Autodesk Inventor part; units mm, degrees
ref_plane "YZ Plane" through (0, 0, 0) normal (1, 0, 0) x (0, 1, 0)
ref_plane "XZ Plane" through (0, 0, 0) normal (0, 1, 0) x (-1, 0, 0)
ref_plane "XY Plane" through (0, 0, 0) normal (0, 0, 1) x (1, 0, 0)
sketch "スケッチ1" plane through (0, 0, 0) normal (0, 0, 1) x (1, 0, 0)
  line L0 (0, 0) -> (-22, 0)
  line L1 (-22, 0) -> (-22, 94)
  line L2 (-22, 94) -> (0, 94)
  line L3 (0, 94) -> (0, 0)
  dimension "d0" = 22
  dimension "d1" = 94
extrude "押し出し1" add sketch "スケッチ1" along normal blind 1.5
sketch "スケッチ2" plane through (0, 0, 0) normal (0, 0, -1) x (-1, 0, 0)
  line L0 (5, 24.2) -> (5, 94)
  circle A0 centre (2.5, 84) radius 1.6
  line L1 (0, 94) -> (22, 94)
  line L2 (5, 94) -> (0, 94)
  circle A1 centre (2.5, 59) radius 1.6
  circle A2 centre (2.5, 34) radius 1.6
  circle A3 centre (2.5, 9) radius 1.6
  point P0 (0, 0)
  point P1 (2.5, 94)
  dimension "d4" = 3.2
  dimension "d5" = 10
  dimension "d8" = 25
extrude "押し出し2" cut sketch "スケッチ2" against normal through all
sketch "スケッチ3" plane through (0, 0, 0) normal (0, 0, -1) x (-1, 0, 0)
  line L0 (3.2909, 24.2) -> (5, 24.2)
  line L1 (0, 0) -> (0, 94)
  line L2 (0, 25.2) -> (6, 25.2)
  line L3 (6, 25.2) -> (6, 0)
  line L4 (6, 0) -> (0, 0)
  line L5 (0, 0) -> (0, 25.2)
  line L6 (5, 14.2) -> (5, 24.2)
  line L7 (22, 0) -> (0, 0)
  dimension "d15" = 1
  dimension "d16" = 1
extrude "押し出し3" cut sketch "スケッチ3" against normal through all
properties part number "rail_backcover"
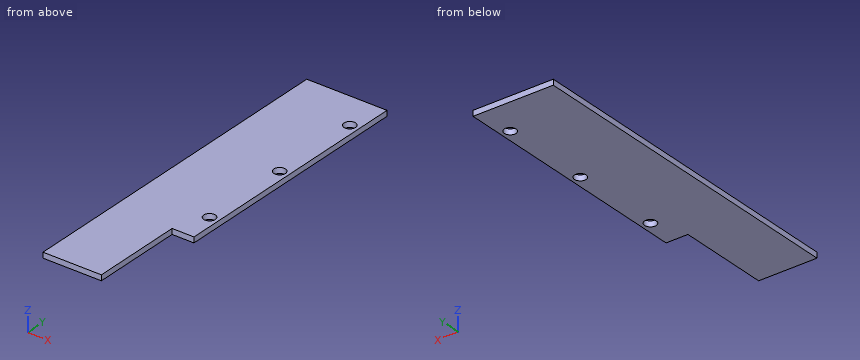
Design review of the part built by this model. Coordinates are the model's own, in mm. Coordinates: 2 decimals unless noted, no trailing zeros. Loops run counter-clockwise (first coordinate to the right, second up) from the corner with the lowest first, then second, coordinate; pieces in that order, holes last. Notation, with made-up numbers: (25.5, -6) -> (73.5, -6) arc R19 ccw to (73.5, 27) -> close; hole circle Ø7 at (-22.5, 8). An arc over 180 degrees is marked (long way). Answer as a JSON object with one key per item and string values.
Q1. Take a section at A-A on y = 84. Give the boundary of the cut face in (x, z), plus the area to 3 significant figures.
Answer block:
{"outline": "(-22, 0) -> (-4.1, 0) -> (-4.1, 1.5) -> (-22, 1.5) -> close; (-0.9, 0) -> (0, 0) -> (0, 1.5) -> (-0.9, 1.5) -> close", "area": "28.2 mm^2"}
Q2. To check wall thickness, follow L1, parallel to Y at x = -2.5, z = 0.45; L2, parallel to Y at x = -3, z = 1.4; L3, parallel to X at y = 12, z = 0.7. State the ranges of each line that lie inside material, in increasing order.
Answer block:
{"L1": "y = 25.2 to 32.4, 35.6 to 57.4, 60.6 to 82.4, 85.6 to 94", "L2": "y = 25.2 to 32.48, 35.52 to 57.48, 60.52 to 82.48, 85.52 to 94", "L3": "x = -22 to -6"}
Q3. Clearance check with a flat-ended pin moving along its axis: pin 1 Ø1.9 at (x, y) = (-2.5, 34) entering from -Z. State where the tip first meets the part, or that it passes through.
Answer block:
{"pin 1": "passes through"}
Q4. Take a section at B-B on z = 0.4. Give the boundary of the cut face in (x, y), plus the area to 3 significant figures.
Answer block:
{"outline": "(-22, 0) -> (-6, 0) -> (-6, 25.2) -> (0, 25.2) -> (0, 94) -> (-22, 94) -> close; hole circle Ø3.2 at (-2.5, 34); hole circle Ø3.2 at (-2.5, 59); hole circle Ø3.2 at (-2.5, 84)", "area": "1,890 mm^2"}
Q5. Take a section at C-C on x = -2.5. Give the boundary of the cut face in (y, z), plus the area to 3 significant figures.
Answer block:
{"outline": "(25.2, 0) -> (32.4, 0) -> (32.4, 1.5) -> (25.2, 1.5) -> close; (35.6, 0) -> (57.4, 0) -> (57.4, 1.5) -> (35.6, 1.5) -> close; (60.6, 0) -> (82.4, 0) -> (82.4, 1.5) -> (60.6, 1.5) -> close; (85.6, 0) -> (94, 0) -> (94, 1.5) -> (85.6, 1.5) -> close", "area": "88.8 mm^2"}
